from build123d import *

# Parameters (mm, degrees)
SKETCH2_W             = 17
SKETCH2_H             = 2.2
BOSS_EXTRUDE1_DEPTH   = 10
BOSS_EXTRUDE1_2_DEPTH = 10
SKETCH2_4_W           = 17
SKETCH2_4_H           = 7
BOSS_EXTRUDE2_DEPTH   = 2
FILLET2_R             = 2


with BuildPart() as part:
    # Sketch2 → Boss-Extrude1 (new body)
    with BuildSketch(Plane.XY):
        with Locations((8.5, 2.4)):
            Rectangle(SKETCH2_W, SKETCH2_H)
    extrude(amount=BOSS_EXTRUDE1_DEPTH)



with BuildPart() as body_2:
    # Sketch2 → Boss-Extrude1 2 (new body)
    with BuildSketch(Plane.XY):
        with BuildLine():
            Line((1.215476742, -0.4), (0, -0.4))
            Line((0, -0.4), (0, -3.5))
            Line((0, -3.5), (17, -3.5))
            Line((17, -3.5), (17, -0.4))
            Line((17, -0.4), (13.784523258, -0.4))
            ThreePointArc((13.784523258, -0.4), (12.5, -1.9), (11.215476742, -0.4))
            Line((11.215476742, -0.4), (8.784523258, -0.4))
            ThreePointArc((8.784523258, -0.4), (7.5, -1.9), (6.215476742, -0.4))
            Line((6.215476742, -0.4), (3.784523258, -0.4))
            ThreePointArc((3.784523258, -0.4), (2.5, -1.9), (1.215476742, -0.4))
        make_face()
    extrude(amount=BOSS_EXTRUDE1_2_DEPTH)


with BuildPart() as part_1:
    add(part.part)

    add(body_2.part)  # Boss-Extrude2 merges body 2
    # Sketch2<4> → Boss-Extrude2 (add)
    with BuildSketch(Plane.XY):
        with Locations((8.5, 0)):
            Rectangle(SKETCH2_4_W, SKETCH2_4_H)
    extrude(amount=-BOSS_EXTRUDE2_DEPTH)

    # Mirror1: part across plane


with BuildPart() as part_2:
    add(part_1.part)
    add(part_1.part.mirror(Plane(origin=(17, 0, 10), x_dir=(0, 0, 1), z_dir=(-1, 0, 0))))

    # Fillet2
    # the kernel refuses this fillet: 2 mm, written as the material it takes off along each edge
    with BuildSketch(Plane(origin=(-5, -3.5, 10), x_dir=(0, 0, -1), z_dir=(1, 0, 0)), Plane(origin=(-5, 3.5, -2), x_dir=(0, 0, 1), z_dir=(1, 0, 0)), Plane(origin=(-5, -3.5, -2), x_dir=(0, 1, 0), z_dir=(1, 0, 0))) as fillet2_piece_1:
        with BuildLine():
            CenterArc((FILLET2_R, FILLET2_R), FILLET2_R, 180, 90)
            Line((0, FILLET2_R), (0, 0))
            Line((0, 0), (FILLET2_R, 0))
        make_face()
    extrude(amount=44, mode=Mode.SUBTRACT)
    with BuildSketch(Plane(origin=(39, 3.5, 10), x_dir=(0, -1, 0), z_dir=(-1, 0, 0))) as fillet2_piece_2:
        with BuildLine():
            CenterArc((FILLET2_R, -FILLET2_R), FILLET2_R, 90, 90)
            Line((0, -FILLET2_R), (0, 0))
            Line((0, 0), (FILLET2_R, 0))
        make_face()
    extrude(amount=44, mode=Mode.SUBTRACT)


solid = part_2.part
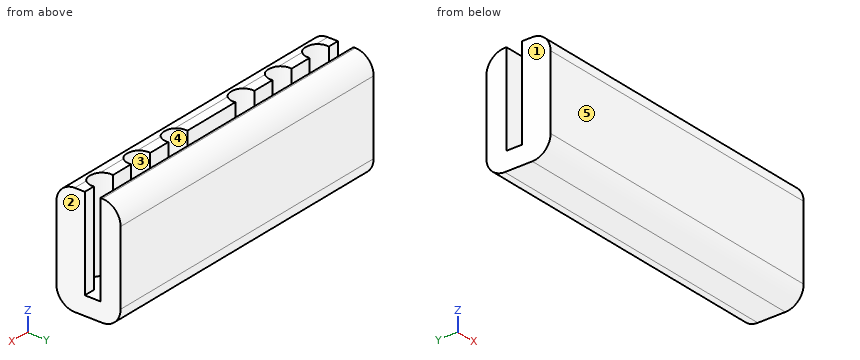
Can you work these out from the model? Positions are in its coordinate system, mm. Face numbers are marked on the shaded views. A direction names the side the tool comes from. Coordinates: 2 decimals unless noted, no trailing zeros. Order: outer loops, then holes, each group sorted by start corner. A loop starts at its lowest first (then second) coordinate and runs counter-clockwise, first axis right, second up. Notation, with made-up numbers: M 80,89 L 115,89 A18 ccw 115,112 Z; hole C 39,-35 d8. An arc over 180 degrees is marked long. Answer as CSV lines item,"result".
(1) Suppose I cut it at D-D on x = 32. Please give me the cut outline in (y, z), plus the area to 3 significant figures.
Geometry check:
outline,"M -3.5,0 A2 ccw -1.5,-2 L 1.5,-2 A2 ccw 3.5,0 L 3.5,8 A2 ccw 1.5,10 L 1.3,10 L 1.3,0 L -1.8,0 L -1.8,9.98 A2 ccw -3.5,8 Z"
area,"49.6 mm^2"
(2) Suppose I cut it at B-B on x = 17.5. Please give me the cut outline in (y, z).
Geometry check:
outline,"M -3.5,0 A2 ccw -1.5,-2 L 1.5,-2 A2 ccw 3.5,0 L 3.5,8 A2 ccw 1.5,10 L 1.3,10 L 1.3,0 L -0.4,0 L -0.4,10 L -1.5,10 A2 ccw -3.5,8 Z"
(3) Please list where these lines run through material, in increasing order: L1, parallel to Y at x = 26.5, z = 4; L2, parallel to Y at x = 16, z = 2.5; L3, parallel to Z at x = 5.5, y = 0.5.
Geometry check:
L1,"-3.5 to -1.9, 1.3 to 3.5"
L2,"-3.5 to -0.4, 1.3 to 3.5"
L3,"-2 to 0"
(4) I'm going to push a flat-ended pin straight in: pin 1 (1.6 mm diameter, centred on x = 21.5, y = -0.6, fed in from +Z). Where does the tip first touch, or does it pass through?
Geometry check:
pin 1,"z = 0"
(5) Suppose I cut it at C-C on y = -0.75. Please give me the cut outline in (x, z), plus the area to 3 significant figures.
Geometry check:
outline,"M 0,-2 L 34,-2 L 34,10 L 32.79,10 L 32.79,0 L 30.21,0 L 30.21,10 L 27.79,10 L 27.79,0 L 25.21,0 L 25.21,10 L 22.79,10 L 22.79,0 L 20.21,0 L 20.21,10 L 13.79,10 L 13.79,0 L 11.21,0 L 11.21,10 L 8.79,10 L 8.79,0 L 6.21,0 L 6.21,10 L 3.79,10 L 3.79,0 L 1.21,0 L 1.21,10 L 0,10 Z"
area,"253 mm^2"
(6) Suppose I cut it at A-A on z = 3.75. Please give me the cut outline in (x, y), plus the area to 3 significant figures.
Geometry check:
outline,"M 0,-3.5 L 34,-3.5 L 34,-0.4 L 32.78,-0.4 A1.3 cw long 30.22,-0.4 L 27.78,-0.4 A1.3 cw long 25.22,-0.4 L 22.78,-0.4 A1.3 cw long 20.22,-0.4 L 13.78,-0.4 A1.3 cw long 11.22,-0.4 L 8.78,-0.4 A1.3 cw long 6.22,-0.4 L 3.78,-0.4 A1.3 cw long 1.22,-0.4 L 0,-0.4 Z; M 0,1.3 L 34,1.3 L 34,3.5 L 0,3.5 Z"
area,"161 mm^2"
(7) On a 3-axis mill with a long thin cutter (end or side, diameter ignored), from which of +Z, -Z, +X, -X, +Y, -Y can I reach the whole of each face in a straight line? I mean the marked faces 4 and 5. Say none if no direction works.
Geometry check:
face 4,"+Z"
face 5,"+Z, -Z, +X, -X, -Y"
(8) If we mould it in two halves opening along X, with no side actions, what happens to the marked faces 1, 2 and 3? For each: released by +X, released by -X, zero draft, split by the parting line, or undercut.
Geometry check:
face 1,"released by -X"
face 2,"released by +X"
face 3,"undercut"
